Verification items for the finished model (mm, model axes). A direction names the side the tool comes from. Coordinates: 2 decimals unless noted, no trailing zeros. Loops run counter-clockwise (first coordinate to the right, second up) from the corner with the lowest first, then second, coordinate; pieces in that order, holes last. Notation, with made-up numbers: (11.25, -35) -> (32.25, -35) arc R24 ccw to (32.25, -15) -> close; hole circle Ø7 at (84.5, 70.25). An arc over 180 degrees is marked (long way). Write item = value, one per line.
```python
from build123d import *

# Parameters (mm, degrees)
F0_W           = 76.9891291857
F0_H           = 47.9887388647
F0_R           = 11.2733779571
F1_DEPTH       = 50.8
F2_R           = 5.08
F4_D           = 12.7
F4_DEPTH       = 25.4
F4_CBORE_D     = 12.7
F4_CBORE_DEPTH = 6.35
F4_TIP         = 3.8154649308


with BuildPart() as f1:
    # F0 (on Front) → F1 (new body)
    with BuildSketch(Plane.XZ):
        Rectangle(F0_W, F0_H)
        Circle(F0_R, mode=Mode.SUBTRACT)
    extrude(amount=F1_DEPTH)

    # F2
    f2_edges = [f1.edges().sort_by_distance(p)[0] for p in [
        (38.494565, -50.8, 0),
        (-38.494565, -50.8, 0),
        (0, -50.8, 23.994369),
        (0, -50.8, -23.994369),
        (-11.273378, -50.8, 0),
    ]]
    fillet(f2_edges, radius=F2_R)

    # F4
    with Locations(Plane.XY.offset(23.9943694323)):
        with Locations((-21.5776711702, -20.1967004687), (18.2978659868, -17.7800003439)):
            CounterBoreHole(F4_D / 2, F4_CBORE_D / 2, F4_CBORE_DEPTH, depth=F4_DEPTH)
            with Locations((0, 0, -(F4_DEPTH + F4_TIP / 2))):  # 118° drill point
                Cone(0, F4_D / 2, F4_TIP, mode=Mode.SUBTRACT)


solid = f1.part
```
1) Tool access check on faces 1 (the face through (15.368, -23.414, 11.117)), 2 (the face through (38.495, -23, 0)). Record the directions out of +Z, -Z, +X, -X, +Y, -Y that give a thin tool (end or side, any length) a straight path to the whole face; none if there is none.
Ans:
face_1 = +Z
face_2 = +Z, -Z, +X, +Y, -Y
2) Material ranges on line 1 (X direction, y = -17.78, z = 5.75); line 2 (Y direction, x = -22, z = 7); line 3 (X direction, y = -17.5, z = 21), recorded low to high.
Ans:
line_1 = -38.49 to -27.45, -15.71 to -9.7, 9.7 to 11.95, 24.65 to 38.49
line_2 = -50.8 to -26.53, -13.86 to 0
line_3 = -38.49 to -27.33, -15.83 to 11.95, 24.64 to 38.49
3) Depth check by flat-ended pin: pin 1 Ø13.5 at (x, z) = (0, 0) entering from +Y (3 decimals). Enter the tip coordinate at first touch or a pass-through.
Ans:
pin_1 = through
4) Sectioned sample at D-D, the plane z = 21. Record the cut outline in (x, y).
Ans:
outline = (-38.49, -45.72) arc R5.08 ccw to (-35.5, -50.35) -> (35.5, -50.35) arc R5.08 ccw to (38.49, -45.72) -> (38.49, 0) -> (-38.49, 0) -> close; hole circle Ø12.7 at (-21.58, -20.2); hole circle Ø12.7 at (18.3, -17.78)
5) Sectioned sample at A-A, the plane x = 0. Record the cut outline in (y, z), plus the area to 3 significant figures.
Ans:
outline = (-50.8, -18.91) arc R5.08 ccw to (-45.72, -23.99) -> (0, -23.99) -> (0, -11.27) -> (-45.72, -11.27) arc R5.08 ccw to (-50.8, -16.35) -> close; (-50.8, 16.35) arc R5.08 ccw to (-45.72, 11.27) -> (0, 11.27) -> (0, 23.99) -> (-45.72, 23.99) arc R5.08 ccw to (-50.8, 18.91) -> close
area = 1,270 mm2
6) Release check for a two-part mould opening along Y. For faces 3 (the face through (-2.444, -22.54, -11.005)), 4 (the face through (-22.39, -19.45, -4.56)), 5 (the face through (-37.05, -49.27, 0.34)) record: pulls with the +Y half, pulls with the -Y half, needs draft (parallel to the pull), parting line crosses it, or undercut.
Ans:
face_3 = needs draft
face_4 = undercut
face_5 = pulls with the -Y half
7) Sectioned sample at C-C, the plane y = -10. Record the cut outline in (x, z).
Ans:
outline = (-38.49, -23.99) -> (38.49, -23.99) -> (38.49, 23.99) -> (-38.49, 23.99) -> close; hole circle Ø22.55 at (0, 0)
8) Sectioned sample at B-B, the plane z = 0. Record the cut outline in (x, y).
Ans:
outline = (-38.49, -45.72) arc R5.08 ccw to (-33.41, -50.8) -> (-16.35, -50.8) arc R5.08 ccw to (-11.27, -45.72) -> (-11.27, 0) -> (-38.49, 0) -> close; (11.27, -45.72) arc R5.08 ccw to (16.35, -50.8) -> (33.41, -50.8) arc R5.08 ccw to (38.49, -45.72) -> (38.49, 0) -> (11.27, 0) -> close; hole circle Ø12.7 at (-21.58, -20.2); hole circle Ø12.7 at (18.3, -17.78)
